```python
from build123d import *

# Parameters (mm, degrees)
F1_DEPTH = 25.4
F3_DEPTH = 12.7
F5_DEPTH = 25.4
F6_DEPTH = 20.0035


with BuildPart() as f1:
    # F0 (on Front) → F1 (new body)
    with BuildSketch(Plane.XZ):
        Polygon((-50.2629226224, -17.4625), (-50.2629226224, 39.6875), (-52.8029226224, 39.6875), (-52.8029226224, -20.0025), (-37.2403003217, -20.0025), (30.3916713614, -2.54), (55.4690490608, -2.54), (55.4690490608, 0), (30.0690490608, 0), (-37.5629226224, -17.4625), align=None)
    extrude(amount=F1_DEPTH)

    # F3 (add): a face of the model
    f3_faces = [f1.faces().sort_by_distance(p)[0] for p in [
        (42.9303602111, -12.7, -2.54),
    ]]
    extrude(f3_faces, amount=F3_DEPTH)

    # F4 (on face) → F5 (join)
    with BuildSketch(Plane.XZ.offset(25.4)):
        Polygon((27.3174908304, -3.33375), (30.3916713614, -15.24), (30.3916713614, -2.54), align=None)
    extrude(amount=-F5_DEPTH)

    # F2 (on face) → F6 (cut, through all)
    with BuildSketch(Plane.XY):
        with BuildLine():
            Line((42.7690490608, -12.7), (45.5753790986, -9.8936699622))
            ThreePointArc((45.5753790986, -9.8936699622), (42.7690490608, -8.73125), (39.962719023, -9.8936699622))
            Line((39.962719023, -9.8936699622), (42.7690490608, -12.7))
        make_face()
        with BuildLine():
            ThreePointArc((45.5753790986, -15.5063300378), (46.4356959554, -14.2187748722), (46.7377990608, -12.7))
            ThreePointArc((46.7377990608, -12.7), (46.4356959554, -11.1812251278), (45.5753790986, -9.8936699622))
            Line((45.5753790986, -9.8936699622), (42.7690490608, -12.7))
            Line((42.7690490608, -12.7), (45.5753790986, -15.5063300378))
        make_face()
        with BuildLine():
            ThreePointArc((39.962719023, -15.5063300378), (42.7690490608, -16.66875), (45.5753790986, -15.5063300378))
            Line((45.5753790986, -15.5063300378), (42.7690490608, -12.7))
            Line((42.7690490608, -12.7), (39.962719023, -15.5063300378))
        make_face()
        with BuildLine():
            Line((42.7690490608, -12.7), (39.962719023, -9.8936699622))
            ThreePointArc((39.962719023, -9.8936699622), (38.8002990608, -12.7), (39.962719023, -15.5063300378))
            Line((39.962719023, -15.5063300378), (42.7690490608, -12.7))
        make_face()
        with BuildLine():
            ThreePointArc((51.0651573617, -4.4038916991), (49.3692304778, -4.3915855299), (49.3815366471, -6.0875124137))
            Line((49.3815366471, -6.0875124137), (51.0651573617, -4.4038916991))
        make_face()
        with BuildLine():
            Line((51.0651573617, -4.4038916991), (49.3815366471, -6.0875124137))
            ThreePointArc((49.3815366471, -6.0875124137), (50.6747316424, -6.3301435284), (51.4017544892, -5.2334845412))
            ThreePointArc((51.4017544892, -5.2334845412), (51.314400722, -4.7858457611), (51.0651573617, -4.4038916991))
        make_face()
        with BuildLine():
            ThreePointArc((51.4017544892, -20.0924845412), (50.6505107302, -18.9858987941), (49.3447978224, -19.2757487616))
            Line((49.3447978224, -19.2757487616), (51.0278652688, -20.958816208))
            ThreePointArc((51.0278652688, -20.958816208), (51.3042932299, -20.564269372), (51.4017544892, -20.0924845412))
        make_face()
        with BuildLine():
            Line((51.0278652688, -20.958816208), (49.3447978224, -19.2757487616))
            ThreePointArc((49.3447978224, -19.2757487616), (49.3692304778, -20.9343835526), (51.0278652688, -20.958816208))
        make_face()
        with BuildLine():
            ThreePointArc((36.5427544892, -20.0924845412), (36.455400722, -19.6448457611), (36.2061573617, -19.2628916991))
            Line((36.2061573617, -19.2628916991), (34.5225366471, -20.9465124137))
            ThreePointArc((34.5225366471, -20.9465124137), (35.8157316424, -21.1891435284), (36.5427544892, -20.0924845412))
        make_face()
        with BuildLine():
            Line((34.5225366471, -20.9465124137), (36.2061573617, -19.2628916991))
            ThreePointArc((36.2061573617, -19.2628916991), (34.5102304778, -19.2505855299), (34.5225366471, -20.9465124137))
        make_face()
        with BuildLine():
            ThreePointArc((34.4857978224, -4.4167487616), (34.5102304778, -6.0753835526), (36.1688652688, -6.099816208))
            Line((36.1688652688, -6.099816208), (34.4857978224, -4.4167487616))
        make_face()
        with BuildLine():
            Line((34.4857978224, -4.4167487616), (36.1688652688, -6.099816208))
            ThreePointArc((36.1688652688, -6.099816208), (36.4452932299, -5.705269372), (36.5427544892, -5.2334845412))
            ThreePointArc((36.5427544892, -5.2334845412), (35.7915107302, -4.1268987941), (34.4857978224, -4.4167487616))
        make_face()
    extrude(amount=-F6_DEPTH, mode=Mode.SUBTRACT)


solid = f1.part
```
Input: part model. Units: mm. Frame: model coordinates. A direction names the side the tool comes from. Round coordinates to 2 decimals unless told otherwise and drop trailing zeros. Loops run counter-clockwise (first coordinate to the right, second up) from the corner with the lowest first, then second, coordinate; pieces in that order, holes last.
1) Set-up query: faces 4 (the flat face through (5, 0, -8)), 5 (the flat face through (-3.27, -12.52, -8.61)), 6 (the flat face through (-5.413, -12.522, -11.785)), 7 (the flat face through (46, -10, 0)). Return all of +Z, -Z, +X, -X, +Y, -Y with unobstructed straight access to the full face (end or side cutting, diameter ignored); none if empty.
Ans:
face 4: +Z, -Z, +X, -X, +Y
face 5: +Z, +Y, -Y
face 6: -Z, +Y, -Y
face 7: +Z, +X, +Y, -Y
2) Material intervals for line 1 (X direction, y = -2, z = 3); line 2 (Z direction, x = 32.5, y = -23.5); line 3 (Z direction, x = -46.5, y = -18), sorted ascending.
Ans:
line 1: x = -52.8 to -50.26
line 2: z = -15.24 to 0
line 3: z = -20 to -17.46
3) Section query C-C on y = -23. Return the cut outline in (x, z), plus the area to 3 significant figures.
Ans:
outline: (-52.8, -20) - (-37.24, -20) - (27.32, -3.33) - (30.39, -15.24) - (55.47, -15.24) - (55.47, 0) - (30.07, 0) - (-37.56, -17.46) - (-50.26, -17.46) - (-50.26, 39.69) - (-52.8, 39.69) - close
area: 764 mm2
4) Pin query (flat end, axial travel): pin 1 (6 mm diameter, centred on x = 17.5, y = -10, fed in from -Z); pin 2 (1 mm diameter, centred on x = 34.5, y = -19.5, fed in from +Z); pin 3 (1 mm diameter, centred on y = -7, z = 26, fed in from +X). Return the tip coordinate at first contact, or that it passes through.
Ans:
pin 1: stops at z = -6.64
pin 2: stops at z = 0
pin 3: stops at x = -50.26
5) Section query B-B on z = -2. Return the cut outline in (x, y), plus the area to 3 significant figures.
Ans:
outline: (-52.8, -25.4) - (-50.26, -25.4) - (-50.26, 0) - (-52.8, 0) - close; (22.32, -25.4) - (55.47, -25.4) - (55.47, 0) - (22.32, 0) - close; hole circle Ø2.38 at (35.35, -20.09); hole circle Ø2.38 at (35.35, -5.23); hole circle Ø7.94 at (42.77, -12.7); hole circle Ø2.38 at (50.21, -20.09); hole circle Ø2.38 at (50.21, -5.23)
area: 839 mm2
6) Section query A-A on z = -12. Return the cut outline in (x, y), plus the area to 3 significant figures.
Ans:
outline: (-52.8, -25.4) - (-50.26, -25.4) - (-50.26, 0) - (-52.8, 0) - close; (-16.41, -25.4) - (-6.25, -25.4) - (-6.25, 0) - (-16.41, 0) - close; (29.56, -25.4) - (55.47, -25.4) - (55.47, 0) - (29.56, 0) - close; hole circle Ø2.38 at (35.35, -20.09); hole circle Ø2.38 at (35.35, -5.23); hole circle Ø7.94 at (42.77, -12.7); hole circle Ø2.38 at (50.21, -20.09); hole circle Ø2.38 at (50.21, -5.23)
area: 913 mm2
7) Section query D-D on y = -11.5. Return the cut outline in (x, z), plus the area to 3 significant figures.
Ans:
outline: (-52.8, -20) - (-37.24, -20) - (27.32, -3.33) - (30.39, -15.24) - (38.99, -15.24) - (38.99, 0) - (30.07, 0) - (-37.56, -17.46) - (-50.26, -17.46) - (-50.26, 39.69) - (-52.8, 39.69) - close; (46.55, -15.24) - (55.47, -15.24) - (55.47, 0) - (46.55, 0) - close
area: 649 mm2
8) Pull-direction query (X, two-part tool) for faces 1 (the flat face through (28.833, -12.878, -9.204)), 2 (the flat face through (46, -10, -15.24)), 3 (the flat face through (-52.803, -13, 10)); classes: released by +X, released by -X, zero draft, split by the parting line, or undercut.
Ans:
face 1: undercut
face 2: zero draft
face 3: released by -X
